The drawing under review shows one solid part. Ordinate dimensions are in mm from its lowest x, y, z. A direction names the side the tool comes from. Round coordinates to 2 decimals unless told otherwise and drop trailing zeros. Write each loop counter-clockwise with the first axis right and the second up, starting at its lowest first coordinate (ties: lowest second). Pieces come first, ordered by that corner, then holes. Notation, with made-up numbers: (57, 69) -> (95, 69) arc R20 cw to (95, 102) -> close; hole circle Ø3 at (-11.75, 58). An arc over 180 degrees is marked (long way). Write item = value, one per line. Start each with the question number.
Item 1: For pin 1 Ø1 at (x, y) = (12.5, 186.5) entering from +Z (3 decimals); pin 2 Ø3 at (y, z) = (223.5, 7.5) entering from -X (3 decimals); pin 3 Ø4 at (x, y) = (8.5, 230) entering from -Z, all flat-tipped, find the tip position at first contact; note any pin that passes through.
Item 2: Add section B-B, the plane x = 32. State the section outline as (y, z) points (3 decimals).
Item 3: Add section C-C, the plane z = 6.5. State the section outline as (x, y) points (3 decimals).
Item 4: To check wall thickness, follow L1, parallel to X at y = 74, z = 35 (3 decimals); L2, parallel to Z at x = 34, y = 300.5 (3 decimals). State the ranges of each line that lie inside material, in increasing order.
Item 5: Machinability: for the marked faces 1 and 2, which of the approach directions +Z, -Z, +X, -X, +Y, -Y give a long, thin tool a straight path to every point of the face, cutting with its end or side? Answer none if there is none.
Item 6: Add section A-A, the plane y = 73. State the section outline as (x, z) points (3 decimals), then the cut area to 3 significant figures.
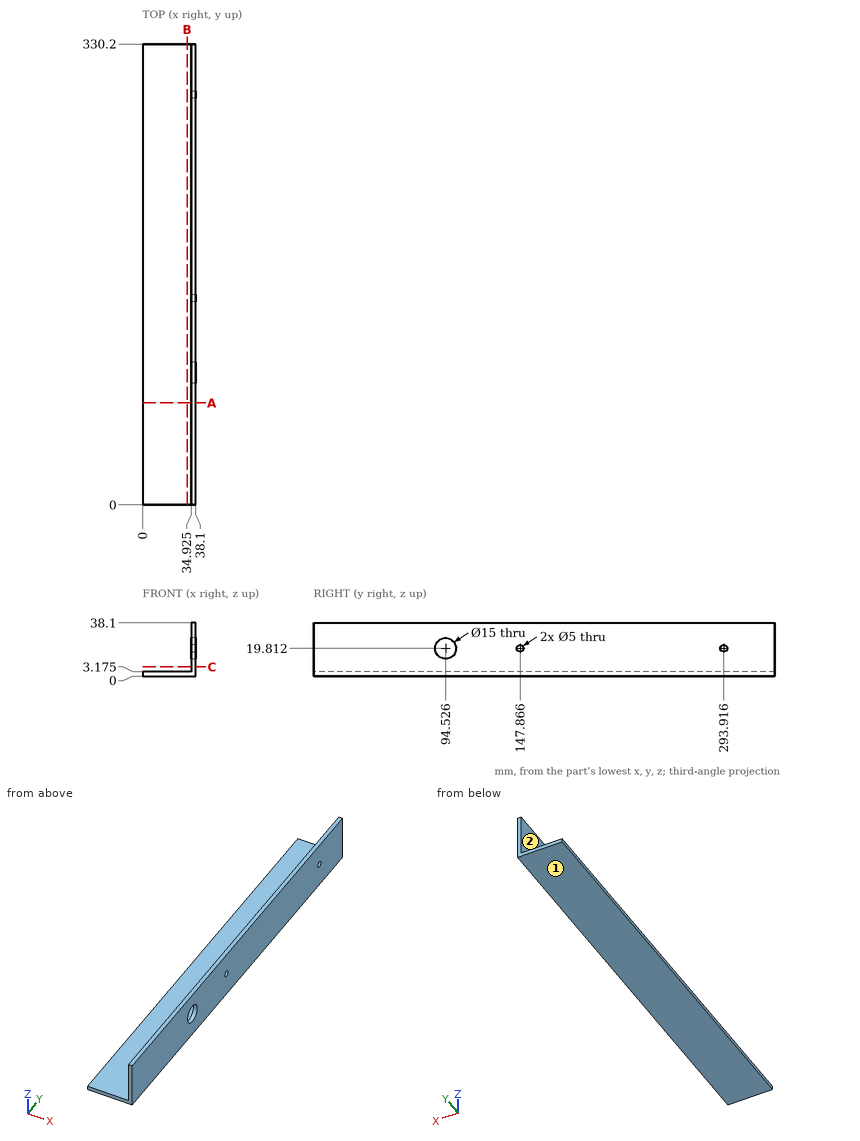
Result set:
q1.pin_1 = 3.175
q1.pin_2 = 34.925
q1.pin_3 = 0
q2.outline = (0, 0) -> (330.2, 0) -> (330.2, 3.175) -> (0, 3.175) -> close
q3.outline = (34.925, 0) -> (38.1, 0) -> (38.1, 330.2) -> (34.925, 330.2) -> close
q4.L1 = 34.925 to 38.1
q4.L2 = 0 to 3.175
q5.face_1 = -Z, +X, -X, +Y, -Y
q5.face_2 = +Z, -X, +Y, -Y
q6.outline = (0, 0) -> (38.1, 0) -> (38.1, 38.1) -> (34.925, 38.1) -> (34.925, 3.175) -> (0, 3.175) -> close
q6.area = 232 mm²
